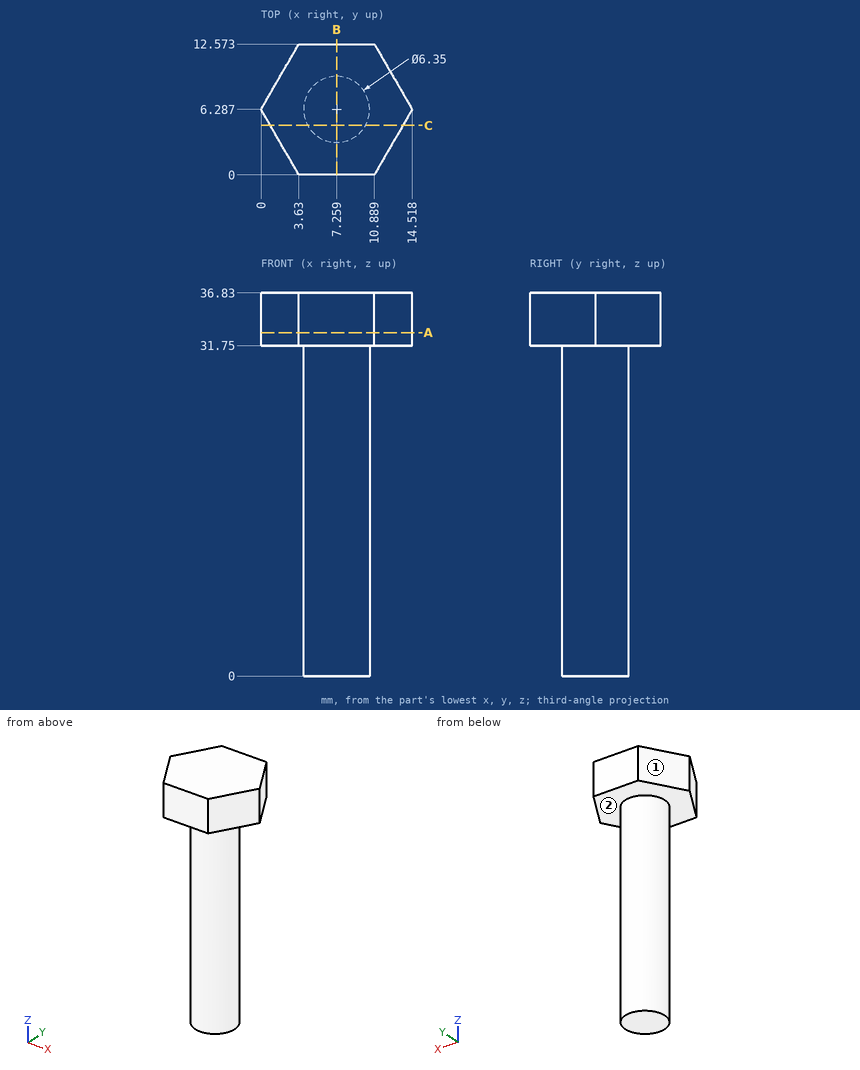
Here's the drawing with two shaded views (mm, measured from the low corner). I have some questions. A direction names the side the tool comes from. Give positions to 0.01 mm unless a question says otherwise; leave off trailing zeros. Loops run counter-clockwise (first coordinate to the right, second up) from the corner with the lowest first, then second, coordinate; pieces in that order, holes last. Notation, with made-up numbers: M 72,79 L 91,79 A12 ccw 91,86 Z; hole C 62,-31.75 d8. An arc over 180 degrees is marked long. One line per item, written item: value.
1) Imagine slicing it at B-B on x = 7.25. Write out the boundary of the cut face in (y, z).
Geometry check:
outline: M 0,31.75 L 3.11,31.75 L 3.11,0 L 9.46,0 L 9.46,31.75 L 12.57,31.75 L 12.57,36.83 L 0,36.83 Z
2) I'm going to push flat-ended pins straight in: pin 1 (1.5 mm diameter, centred on x = 4, y = 9, fed in from -Z); pin 2 (4 mm diameter, centred on y = 10, z = 31.5, fed in from -X); pin 3 (4 mm diameter, centred on y = 5, z = 16, fed in from -X). Where does each tip first touch, or does it pass through?
Geometry check:
pin 1: stops at z = 31.75
pin 2: stops at x = 1
pin 3: stops at x = 4.08
3) On a 3-axis mill with a long thin cutter (end or side, diameter ignored), from which of +Z, -Z, +X, -X, +Y, -Y can I reach the whole of each face in a straight line? I mean the marked faces 1 and 2. Say none if no direction works.
Geometry check:
face 1: +Z, -Z, -X, +Y
face 2: -Z
4) Please list where these lines run through material, in increasing order: line 1 (X direction, y = 6.5, z = 31); line 2 (Z direction, x = 3.5, y = 10.5); line 3 (X direction, y = 9, z = 27) (1 decimal).
Geometry check:
line 1: x = 4.09 to 10.43
line 2: z = 31.75 to 36.83
line 3: x = 5.6 to 8.9
5) Imagine slicing it at A-A on z = 33. Write out the boundary of the cut face in (x, y).
Geometry check:
outline: M 0,6.29 L 3.63,0 L 10.89,0 L 14.52,6.29 L 10.89,12.57 L 3.63,12.57 Z
6) Imagine slicing it at C-C on y = 4.75. Write out the boundary of the cut face in (x, z), and give its area (3 significant figures).
Geometry check:
outline: M 0.89,31.75 L 4.48,31.75 L 4.48,0 L 10.04,0 L 10.04,31.75 L 13.63,31.75 L 13.63,36.83 L 0.89,36.83 Z
area: 241 mm²
